```python
from build123d import *

# Parameters (mm, degrees)
F0_W         = 57.0548474789
F0_H         = 99.3303954601
F1_DEPTH     = 30
F0_W_2       = 75.9585499763
F0_H_2       = 127.8578191996
F2_DEPTH     = 10
F3_C1_SIZE2  = 3
F3_C1_SIZE   = 17.0138454589
F3_C2_SIZE2  = 3
F3_C2_SIZE   = 17.0138454589
F3_C3_SIZE2  = 3
F3_C3_SIZE   = 17.0138454589
F3_C4_SIZE2  = 3
F3_C4_SIZE   = 17.0138454589
F4_T4_DEPTH  = 57.0548474789
F4_T9_DEPTH  = 99.3303954601
F4_T14_DEPTH = 57.0548474789
F4_T19_DEPTH = 99.3303954601
F4_T25_DEPTH = 114.1873722104
F4_T31_DEPTH = 71.9118242292
F4_T40_DEPTH = 114.1873722104
F4_T46_DEPTH = 71.9118242292
F4_T55_DEPTH = 71.9118242292
F4_T61_DEPTH = 114.1873722104
F4_T70_DEPTH = 71.9118242292
F4_T76_DEPTH = 114.1873722104
F4_T81_DEPTH = 157.5717727001
F4_T83_DEPTH = 105.6725034769
F0_W_3       = 134.0444982052
F0_H_3       = 180.7882040739
F5_DEPTH     = 3
F7_D         = 20


# Not quite as in the source:
# - a fillet or chamfer that OpenCascade refuses, or shapes differently, is made with other operations: its cross-section is extruded or revolved along the edge and cut away or added


with BuildPart() as f1:
    # F0 (on Front) → F1 (new body)
    with BuildSketch(Plane.XZ):
        Rectangle(F0_W, F0_H)
    extrude(amount=F1_DEPTH)

    # F0 (on Front) → F2 (join)
    with BuildSketch(Plane.XZ):
        Rectangle(F0_W_2, F0_H_2)
        Rectangle(F0_W, F0_H, mode=Mode.SUBTRACT)
    extrude(amount=F2_DEPTH)

    # F3: chamfer of 3 x 17.0138454589 on 4 edges, made by hand

    # F3_c1
    f3_c1_edges = [f1.edges().sort_by_distance(p)[0] for p in [
        (28.5274237394, -30, 0),
    ]]
    f3_c1_side = f1.faces().sort_by_distance((28.5274237394, -29.94, 0))[0]
    chamfer(f3_c1_edges, length=F3_C1_SIZE, length2=F3_C1_SIZE2, reference=f3_c1_side)

    # F3_c2
    f3_c2_edges = [f1.edges().sort_by_distance(p)[0] for p in [
        (-1.5, -30, 49.6651977301),
    ]]
    f3_c2_side = f1.faces().sort_by_distance((-1.5, -29.94, 49.6651977301))[0]
    chamfer(f3_c2_edges, length=F3_C2_SIZE, length2=F3_C2_SIZE2, reference=f3_c2_side)

    # F3_c3
    f3_c3_edges = [f1.edges().sort_by_distance(p)[0] for p in [
        (-28.5274237394, -30, -1.5),
    ]]
    f3_c3_side = f1.faces().sort_by_distance((-28.5274237394, -29.94, -1.5))[0]
    chamfer(f3_c3_edges, length=F3_C3_SIZE, length2=F3_C3_SIZE2, reference=f3_c3_side)

    # F3_c4
    f3_c4_edges = [f1.edges().sort_by_distance(p)[0] for p in [
        (0, -30, -49.6651977301),
    ]]
    f3_c4_side = f1.faces().sort_by_distance((0, -29.94, -49.6651977301))[0]
    chamfer(f3_c4_edges, length=F3_C4_SIZE, length2=F3_C4_SIZE2, reference=f3_c4_side)

    # F4: chamfer of 0.5 x 5.7150261514 on 8 edges, made by hand


with BuildPart() as f4_tool2:
    # F4_s3 → F4_t4 (new body)
    with BuildSketch(Plane.YZ.offset(-28.5274237394)):
        Polygon((-10, 50.1651977301), (-15.7150261514, 49.6651977301), (-10, 49.6651977301), align=None)
    extrude(amount=F4_T4_DEPTH)

    split(bisect_by=Plane(origin=(0, -8.8848294962, 50.3883719921), x_dir=(1, 0, 0), z_dir=(0, 0.1736481777, -0.984807753)), keep=Keep.TOP)


with BuildPart() as f1_1:
    add(f1.part)

    # F4_t1: union F4_tool2
    add(f4_tool2.part)


with BuildPart() as f4_tool7:
    # F4_s8 → F4_t9 (new body)
    with BuildSketch(Plane.XY.offset(49.6651977301)):
        Polygon((28.5274237394, -15.7150261514), (29.0274237394, -10), (28.5274237394, -10), align=None)
    extrude(amount=-F4_T9_DEPTH)

    split(bisect_by=Plane(origin=(29.8879798774, -5.2700572513, 0), x_dir=(0, 0, 1), z_dir=(-0.984807753, 0.1736481777, 0)), keep=Keep.TOP)


with BuildPart() as f1_2:
    add(f1_1.part)

    # F4_t6: union F4_tool7
    add(f4_tool7.part)


with BuildPart() as f4_tool12:
    # F4_s13 → F4_t14 (new body)
    with BuildSketch(Plane.YZ.offset(28.5274237394)):
        Polygon((-15.7150261514, -49.6651977301), (-10, -50.1651977301), (-10, -49.6651977301), align=None)
    extrude(amount=-F4_T14_DEPTH)

    split(bisect_by=Plane(origin=(0, -8.8848294962, -50.3883719921), x_dir=(1, 0, 0), z_dir=(0, 0.1736481777, 0.984807753)), keep=Keep.TOP)


with BuildPart() as f1_3:
    add(f1_2.part)

    # F4_t11: union F4_tool12
    add(f4_tool12.part)


with BuildPart() as f4_tool17:
    # F4_s18 → F4_t19 (new body)
    with BuildSketch(Plane.XY.offset(-49.6651977301)):
        Polygon((-28.5274237394, -15.7150261514), (-29.0274237394, -10), (-28.5274237394, -10), align=None)
    extrude(amount=F4_T19_DEPTH)

    split(bisect_by=Plane(origin=(-29.8879798774, -5.2700572513, 0), x_dir=(0, 0, 1), z_dir=(0.984807753, 0.1736481777, 0)), keep=Keep.TOP)


with BuildPart() as f1_4:
    add(f1_3.part)

    # F4_t16: union F4_tool17
    add(f4_tool17.part)


with BuildPart() as f4_tool23:
    # F4_s24 → F4_t25 (new body)
    with BuildSketch(Plane.XY.offset(-49.6651977301)):
        Polygon((-28.5274237394, -15.7150261514), (-29.0274237394, -10), (-28.5274237394, -10), align=None)
    extrude(amount=F4_T25_DEPTH)

    split(bisect_by=Plane(origin=(-29.8879798774, -5.2700572513, 0), x_dir=(0, 0, 1), z_dir=(0.984807753, 0.1736481777, 0)), keep=Keep.TOP)

    split(bisect_by=Plane.XY.offset(49.6651977301), keep=Keep.TOP)

    split(bisect_by=Plane.XY.offset(63.9289095998), keep=Keep.BOTTOM)


with BuildPart() as f4_tool29:
    # F4_s30 → F4_t31 (new body)
    with BuildSketch(Plane.YZ.offset(-43.3844004897)):
        Polygon((-10, 50.1651977301), (-15.7150261514, 49.6651977301), (-10, 49.6651977301), align=None)
    extrude(amount=F4_T31_DEPTH)

    split(bisect_by=Plane.YZ.offset(-28.5274237394), keep=Keep.BOTTOM)

    split(bisect_by=Plane.YZ.offset(-37.9792749882), keep=Keep.TOP)

    split(bisect_by=Plane(origin=(0, -8.8848294962, 50.3883719921), x_dir=(1, 0, 0), z_dir=(0, 0.1736481777, -0.984807753)), keep=Keep.TOP)


with BuildPart() as f4_tool23_1:
    add(f4_tool23.part)

    # F4_t35: intersect F4_tool29
    add(f4_tool29.part, mode=Mode.INTERSECT)


with BuildPart() as f1_5:
    add(f1_4.part)

    # F4_t21: union F4_tool23
    add(f4_tool23_1.part)


with BuildPart() as f4_tool38:
    # F4_s39 → F4_t40 (new body)
    with BuildSketch(Plane.XY.offset(64.5221744803)):
        Polygon((28.5274237394, -15.7150261514), (29.0274237394, -10), (28.5274237394, -10), align=None)
    extrude(amount=-F4_T40_DEPTH)

    split(bisect_by=Plane.XY.offset(49.6651977301), keep=Keep.TOP)

    split(bisect_by=Plane(origin=(29.8879798774, -5.2700572513, 0), x_dir=(0, 0, 1), z_dir=(-0.984807753, 0.1736481777, 0)), keep=Keep.TOP)

    split(bisect_by=Plane.XY.offset(63.9289095998), keep=Keep.BOTTOM)


with BuildPart() as f4_tool44:
    # F4_s45 → F4_t46 (new body)
    with BuildSketch(Plane.YZ.offset(-28.5274237394)):
        Polygon((-10, 50.1651977301), (-15.7150261514, 49.6651977301), (-10, 49.6651977301), align=None)
    extrude(amount=F4_T46_DEPTH)

    split(bisect_by=Plane.YZ.offset(28.5274237394), keep=Keep.TOP)

    split(bisect_by=Plane.YZ.offset(37.9792749882), keep=Keep.BOTTOM)

    split(bisect_by=Plane(origin=(0, -8.8848294962, 50.3883719921), x_dir=(1, 0, 0), z_dir=(0, 0.1736481777, -0.984807753)), keep=Keep.TOP)


with BuildPart() as f4_tool38_1:
    add(f4_tool38.part)

    # F4_t50: intersect F4_tool44
    add(f4_tool44.part, mode=Mode.INTERSECT)


with BuildPart() as f1_6:
    add(f1_5.part)

    # F4_t36: union F4_tool38
    add(f4_tool38_1.part)


with BuildPart() as f4_tool53:
    # F4_s54 → F4_t55 (new body)
    with BuildSketch(Plane.YZ.offset(43.3844004897)):
        Polygon((-15.7150261514, -49.6651977301), (-10, -50.1651977301), (-10, -49.6651977301), align=None)
    extrude(amount=-F4_T55_DEPTH)

    split(bisect_by=Plane(origin=(0, -8.8848294962, -50.3883719921), x_dir=(1, 0, 0), z_dir=(0, 0.1736481777, 0.984807753)), keep=Keep.TOP)

    split(bisect_by=Plane.YZ.offset(28.5274237394), keep=Keep.TOP)

    split(bisect_by=Plane.YZ.offset(37.9792749882), keep=Keep.BOTTOM)


with BuildPart() as f4_tool59:
    # F4_s60 → F4_t61 (new body)
    with BuildSketch(Plane.XY.offset(49.6651977301)):
        Polygon((28.5274237394, -15.7150261514), (29.0274237394, -10), (28.5274237394, -10), align=None)
    extrude(amount=-F4_T61_DEPTH)

    split(bisect_by=Plane.XY.offset(-49.6651977301), keep=Keep.BOTTOM)

    split(bisect_by=Plane(origin=(29.8879798774, -5.2700572513, 0), x_dir=(0, 0, 1), z_dir=(-0.984807753, 0.1736481777, 0)), keep=Keep.TOP)

    split(bisect_by=Plane.XY.offset(-63.9289095998), keep=Keep.TOP)


with BuildPart() as f4_tool53_1:
    add(f4_tool53.part)

    # F4_t65: intersect F4_tool59
    add(f4_tool59.part, mode=Mode.INTERSECT)


with BuildPart() as f1_7:
    add(f1_6.part)

    # F4_t51: union F4_tool53
    add(f4_tool53_1.part)


with BuildPart() as f4_tool68:
    # F4_s69 → F4_t70 (new body)
    with BuildSketch(Plane.YZ.offset(28.5274237394)):
        Polygon((-15.7150261514, -49.6651977301), (-10, -50.1651977301), (-10, -49.6651977301), align=None)
    extrude(amount=-F4_T70_DEPTH)

    split(bisect_by=Plane(origin=(0, -8.8848294962, -50.3883719921), x_dir=(1, 0, 0), z_dir=(0, 0.1736481777, 0.984807753)), keep=Keep.TOP)

    split(bisect_by=Plane.YZ.offset(-28.5274237394), keep=Keep.BOTTOM)

    split(bisect_by=Plane.YZ.offset(-37.9792749882), keep=Keep.TOP)


with BuildPart() as f4_tool74:
    # F4_s75 → F4_t76 (new body)
    with BuildSketch(Plane.XY.offset(-64.5221744803)):
        Polygon((-28.5274237394, -15.7150261514), (-29.0274237394, -10), (-28.5274237394, -10), align=None)
    extrude(amount=F4_T76_DEPTH)

    split(bisect_by=Plane.XY.offset(-49.6651977301), keep=Keep.BOTTOM)

    split(bisect_by=Plane(origin=(-29.8879798774, -5.2700572513, 0), x_dir=(0, 0, 1), z_dir=(0.984807753, 0.1736481777, 0)), keep=Keep.TOP)

    split(bisect_by=Plane.XY.offset(-63.9289095998), keep=Keep.TOP)


with BuildPart() as f4_tool68_1:
    add(f4_tool68.part)

    # F4_t80: intersect F4_tool74
    add(f4_tool74.part, mode=Mode.INTERSECT)


with BuildPart() as f1_8:
    add(f1_7.part)

    # F4_t66: union F4_tool68
    add(f4_tool68_1.part)

    # F4_s82 → F4_t81 (cut)
    with BuildSketch(Plane.XY.offset(-78.7858863501)):
        Polygon((37.4792749882, -10), (37.9792749882, -4.2849738486), (37.9792749882, -10), align=None)
        Polygon((-37.4792749882, -10), (-37.9792749882, -4.2849738486), (-37.9792749882, -10), align=None)
    extrude(amount=F4_T81_DEPTH, mode=Mode.SUBTRACT)

    # F4_s84 → F4_t83 (cut)
    with BuildSketch(Plane.YZ.offset(-52.8362517385)):
        Polygon((-10, 63.4289095998), (-4.2849738486, 63.9289095998), (-10, 63.9289095998), align=None)
        Polygon((-10, -63.4289095998), (-4.2849738486, -63.9289095998), (-10, -63.9289095998), align=None)
    extrude(amount=F4_T83_DEPTH, mode=Mode.SUBTRACT)

    # F0 (on Front) → F5 (join)
    with BuildSketch(Plane.XZ):
        Rectangle(F0_W_3, F0_H_3)
        Rectangle(F0_W_2, F0_H_2, mode=Mode.SUBTRACT)
    extrude(amount=F5_DEPTH)

    # F7 (through all)
    with Locations(Plane(origin=(0, 0, 0), x_dir=(1, 0, 0), z_dir=(0, 1, 0))):
        with Locations((0, 90.1845097542)):
            Hole(F7_D / 2)


solid = f1_8.part
```
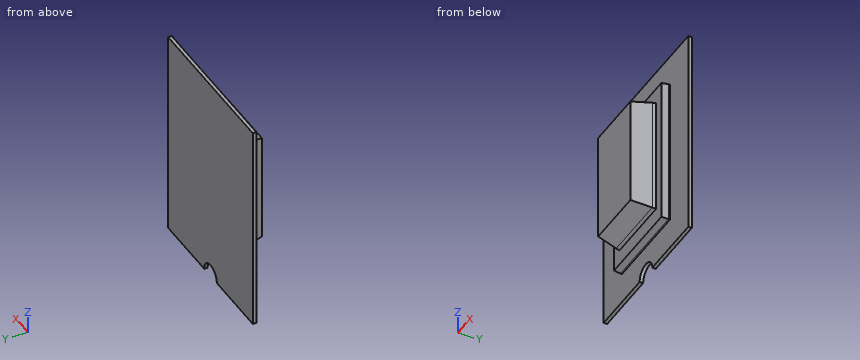
Check sheet for the modelled part. Datum: model origin and axes. Units: mm. Coordinates: 2 decimals unless noted, no trailing zeros. Write each loop counter-clockwise with the first axis right and the second up, starting at its lowest first coordinate (ties: lowest second). Pieces come first, ordered by that corner, then holes. Notation, with made-up numbers: (10, 78) -> (53, 78) arc R35 cw to (53, 110) -> close; hole circle Ø7 at (-31.75, 65.5). An arc over 180 degrees is marked (long way). Use a Markdown table: item, result.
1. Scan lines: line 1 along Y through (x, z) = (53, -82.5); line 2 along Z through (x, y) = (12, -4); line 3 along Y through (x, z) = (-35, -33). Record each from-to range of solid material in increasing order.
Reported:
| item | result |
|---|---|
| line 1 | y = -3 to 0 |
| line 2 | z = -63.93 to 63.93 |
| line 3 | y = -10 to 0 |
2. Sectioned sample at D-D (y = -17). Enter the section's corners in (x, z).
Reported:
| item | result |
|---|---|
| outline | (-27.82, -48.96) -> (27.82, -48.96) -> (27.82, 48.96) -> (-27.82, 48.96) -> close |
3. Sectioned sample at A-A (x = 0). Enter the section's corners in (y, z).
Reported:
| item | result |
|---|---|
| outline | (-30, -46.67) -> (-10.3, -50.14) -> (-10, -50.17) -> (-10, -63.43) -> (-4.28, -63.93) -> (-3, -63.93) -> (-3, -80.18) -> (0, -80.18) -> (0, 90.39) -> (-3, 90.39) -> (-3, 63.93) -> (-4.28, 63.93) -> (-10, 63.43) -> (-10, 50.17) -> (-10.3, 50.14) -> (-30, 46.67) -> close |
4. Go/stop test with flat-tipped pins: pin 1 Ø8 at (x, y) = (-34.5, -25) entering from +Z; pin 2 Ø1 at (x, y) = (3, -4) entering from +Z; pin 3 Ø10 at (x, y) = (27.5, -16.5) entering from -Z; pin 4 Ø0.6 at (y, z) = (-3.5, -11.5) entering from -X. Record where each tip stops, or that it passes through.
Reported:
| item | result |
|---|---|
| pin 1 | passes through |
| pin 2 | stops at z = 63.93 |
| pin 3 | stops at z = -49.93 |
| pin 4 | stops at x = -37.98 |
5. Sectioned sample at C-C (x = 34). Enter the section's corners in (y, z).
Reported:
| item | result |
|---|---|
| outline | (-10, -63.43) -> (-4.28, -63.93) -> (-3, -63.93) -> (-3, -90.39) -> (0, -90.39) -> (0, 90.39) -> (-3, 90.39) -> (-3, 63.93) -> (-4.28, 63.93) -> (-10, 63.43) -> close |
6. Sectioned sample at B-B (z = 7). Enter the section's corners in (x, y).
Reported:
| item | result |
|---|---|
| outline | (-67.02, -3) -> (-37.98, -3) -> (-37.98, -4.28) -> (-37.48, -10) -> (-29.03, -10) -> (-29, -10.3) -> (-25.53, -30) -> (25.53, -30) -> (29, -10.3) -> (29.03, -10) -> (37.48, -10) -> (37.98, -4.28) -> (37.98, -3) -> (67.02, -3) -> (67.02, 0) -> (-67.02, 0) -> close |
